Check sheet for the modelled part. Datum: model origin and axes. Units: mm. Round coordinates to 2 decimals unless told otherwise and drop trailing zeros. Write each loop counter-clockwise with the first axis right and the second up, starting at its lowest first coordinate (ties: lowest second). Pieces come first, ordered by that corner, then holes. Notation, with made-up numbers: M -13,-16 L 6,-16 A7 ccw 6,-4 Z; hole C -39,-14 d2. An arc over 180 degrees is marked long. Answer in a Markdown table with one row per item.
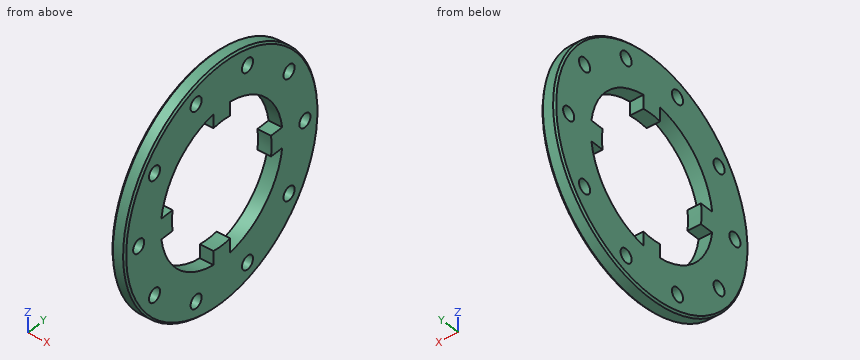
```python
from build123d import *

# Parameters (mm, degrees)
ESQUISSE1_W             = 4
ESQUISSE1_H             = 17
ENL_V_MAT_EXTRU_1_DEPTH = 50.658836072
CHANFREIN1_SIZE         = 0.5
ESQUISSE3_R             = 2
ENL_V_MAT_EXTRU_2_DEPTH = 50.658836072


with BuildPart() as part:
    # Esquisse1 → Base-Révolution (revolve)
    with BuildSketch(Plane.XY, mode=Mode.PRIVATE) as base_r_volution_sk:
        with Locations((2, 26.5)):
            Rectangle(ESQUISSE1_W, ESQUISSE1_H)
    revolve(base_r_volution_sk.sketch.rotate(Axis((0, 0, 0), (1, 0, 0)), 90), axis=Axis((0, 0, 0), (1, 0, 0)))

    # Esquisse2 → Enlèv. mat.-Extru.1 (cut, through all)
    with BuildSketch(Plane.ZY):
        with BuildLine():
            Line((-3, 16), (-3, 21.794494718))
            ThreePointArc((-3, 21.794494718), (-15.556349186, 15.556349186), (-21.794494718, 3))
            Line((-21.794494718, 3), (-16, 3))
            Line((-16, 3), (-16, -3))
            Line((-16, -3), (-21.794494718, -3))
            ThreePointArc((-21.794494718, -3), (-15.556349186, -15.556349186), (-3, -21.794494718))
            Line((-3, -21.794494718), (-3, -16))
            Line((-3, -16), (3, -16))
            Line((3, -16), (3, -21.794494718))
            ThreePointArc((3, -21.794494718), (15.556349186, -15.556349186), (21.794494718, -3))
            Line((21.794494718, -3), (16, -3))
            Line((16, -3), (16, 3))
            Line((16, 3), (21.794494718, 3))
            ThreePointArc((21.794494718, 3), (15.556349186, 15.556349186), (3, 21.794494718))
            Line((3, 21.794494718), (3, 16))
            Line((3, 16), (-3, 16))
        make_face()
    extrude(amount=-ENL_V_MAT_EXTRU_1_DEPTH, mode=Mode.SUBTRACT)

    # Chanfrein1
    chanfrein1_edges = [part.edges().sort_by_distance(p)[0] for p in [
        (0, 0, -35),
        (4, 0, -35),
    ]]
    chamfer(chanfrein1_edges, length=CHANFREIN1_SIZE)

    # Esquisse3 → Enlèv. mat.-Extru.2 (cut, through all)
    with BuildSketch(Plane.ZY):
        with Locations((0, 30)):
            Circle(ESQUISSE3_R)
        with Locations((17.633557569, 24.270509831)):
            Circle(ESQUISSE3_R)
        with Locations((28.531695489, 9.270509831)):
            Circle(ESQUISSE3_R)
        with Locations((28.531695489, -9.270509831)):
            Circle(ESQUISSE3_R)
        with Locations((17.633557569, -24.270509831)):
            Circle(ESQUISSE3_R)
        with Locations((0, -30)):
            Circle(ESQUISSE3_R)
        with Locations((-17.633557569, -24.270509831)):
            Circle(ESQUISSE3_R)
        with Locations((-28.531695489, -9.270509831)):
            Circle(ESQUISSE3_R)
        with Locations((-28.531695489, 9.270509831)):
            Circle(ESQUISSE3_R)
        with Locations((-17.633557569, 24.270509831)):
            Circle(ESQUISSE3_R)
    extrude(amount=-ENL_V_MAT_EXTRU_2_DEPTH, mode=Mode.SUBTRACT)


solid = part.part
```
1. Section check B-B, the plane z = 0. Record the cut outline in (x, y).
Found:
| item | result |
|---|---|
| outline | M 0,-34.5 L 0.5,-35 L 3.5,-35 L 4,-34.5 L 4,-32 L 0,-32 Z; M 0,-28 L 4,-28 L 4,-18 L 0,-18 Z; M 0,18 L 4,18 L 4,28 L 0,28 Z; M 0,32 L 4,32 L 4,34.5 L 3.5,35 L 0.5,35 L 0,34.5 Z |
2. Go/stop test with flat-tipped pins: pin 1 (1.5 mm diameter, centred on x = 1.5, z = 6.5, fed in from -Y); pin 2 (6.5 mm diameter, centred on y = 9.27, z = 28.53, fed in from -X); pin 3 (1.2 mm diameter, centred on x = 1, z = -19, fed in from +Y); pin 4 (3.5 mm diameter, centred on y = -30, z = 0, fed in from +X). Record where each tip stops, or that it passes through.
Found:
| item | result |
|---|---|
| pin 1 | stops at y = -34.52 |
| pin 2 | stops at x = 0 |
| pin 3 | stops at y = 29.77 |
| pin 4 | passes through |
3. Section check C-C, the plane x = 2. Count the separate pieces of the cut face and the enclosed holes in it, and give its area (3 significant figures).
Found:
| item | result |
|---|---|
| separate pieces | 1 |
| enclosed holes | 11 |
| area | 2,300 mm2 |
4. Scan lines: L1, parallel to Y at x = 3.25, z = 0; L2, parallel to Y at x = 0.65, z = -1; L3, parallel to Y at x = 0.7, z = 27. Record each from-to range of solid material in increasing order.
Found:
| item | result |
|---|---|
| L1 | y = -35 to -32, -28 to -18, 18 to 28, 32 to 35 |
| L2 | y = -34.99 to -31.73, -28.27 to -17.97, 17.97 to 28.27, 31.73 to 34.99 |
| L3 | y = -22.27 to -10.56, -7.98 to 7.98, 10.56 to 22.27 |
5. Section check A-A, the plane y = 0. Record the cut outline in (x, z), and give its area (4 significant figures).
Found:
| item | result |
|---|---|
| outline | M 0,-34.5 L 0.5,-35 L 3.5,-35 L 4,-34.5 L 4,-18 L 0,-18 Z; M 0,18 L 4,18 L 4,34.5 L 3.5,35 L 0.5,35 L 0,34.5 Z |
| area | 135.5 mm2 |
